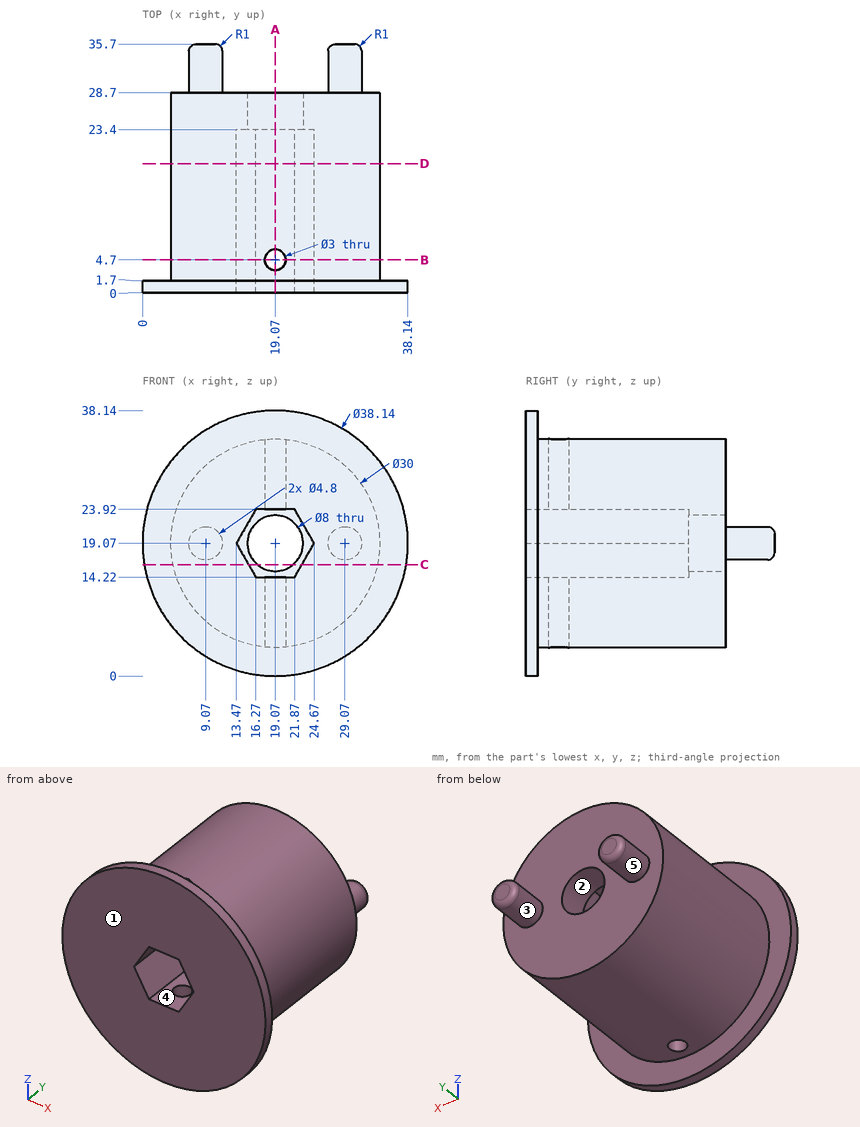
Study the drawing (mm; zero at the part's minimum x, y, z) and answer. A direction names the side the tool comes from. Give positions to 0.01 mm unless a question says otherwise; leave off trailing zeros. Write each loop counter-clockwise with the first axis right and the second up, starting at its lowest first coordinate (ties: lowest second). Pieces come first, ordered by that corner, then holes. Notation, with made-up numbers: (-40, -2) - (-8, -2) arc R27 ccw to (-8, 25) - close; hole circle Ø4 at (49, 26.25). An arc over 180 degrees is marked (long way). Use a Markdown table: item, result.
1. Find the intervals of material crossed by probe 1 along Y at (x, z) = (19, 9); probe 2 along Z at (x, y) = (18.5, 17); probe 3 along Y at (x, z) = (31, 22), in increasing order. Write a range as from..to.
Values follow:
| item | result |
|---|---|
| probe 1 | y = 0..3.2, 6.2..28.7 |
| probe 2 | z = 4.08..14.22, 23.92..34.06 |
| probe 3 | y = 0..28.7 |
2. Section C-C on z = 16 is taken. Write down the section's boundary in (x, y).
Values follow:
| item | result |
|---|---|
| outline | (0.25, 0) - (15.24, 0) - (15.24, 23.4) - (16.51, 23.4) - (16.51, 28.7) - (4.39, 28.7) - (4.39, 1.7) - (0.25, 1.7) - close; (21.63, 23.4) - (22.9, 23.4) - (22.9, 0) - (37.89, 0) - (37.89, 1.7) - (33.75, 1.7) - (33.75, 28.7) - (21.63, 28.7) - close |
3. Section A-A on x = 19.07 is taken. Write down the section's boundary in (y, z).
Values follow:
| item | result |
|---|---|
| outline | (0, 0) - (1.7, 0) - (1.7, 4.07) - (3.2, 4.07) - (3.2, 14.22) - (0, 14.22) - close; (0, 23.92) - (3.2, 23.92) - (3.2, 34.07) - (1.7, 34.07) - (1.7, 38.14) - (0, 38.14) - close; (6.2, 4.07) - (28.7, 4.07) - (28.7, 15.07) - (23.4, 15.07) - (23.4, 14.22) - (6.2, 14.22) - close; (6.2, 23.92) - (23.4, 23.92) - (23.4, 23.07) - (28.7, 23.07) - (28.7, 34.07) - (6.2, 34.07) - close |
4. Each of these flat-tipped pins is pushed along its axis until it touches: P1, Ø10, axis at x = 33, z = 30, coming from the -Y side; P2, Ø1.7, axis at x = 17.5, y = 11, coming from the -Z side; P3, Ø2.5, axis at x = 19.07, y = 4.7, coming from the -Z side; P4, Ø6, axis at x = 19.5, y = 29.5, coming from the +Z side. Where does it stop, or does it pass through?
Values follow:
| item | result |
|---|---|
| P1 | stops at y = 0 |
| P2 | stops at z = 4.09 |
| P3 | passes through |
| P4 | stops at z = 34.07 |
5. For a pull along Z with two mould halves and no side action, classify the marked faces 1, 2 and 3 as released by +Z, released by -Z, zero draft, split by the parting line, or undercut.
Values follow:
| item | result |
|---|---|
| face 1 | zero draft |
| face 2 | undercut |
| face 3 | split by the parting line |
6. Section B-B on y = 4.7 is taken. Write down the section's boundary in (x, z) (1 decimal), plus the area to 3 significant figures.
Values follow:
| item | result |
|---|---|
| outline | (13.5, 19.1) - (16.3, 23.9) - (17.6, 23.9) - (17.6, 34) arc R15 ccw to (17.6, 4.1) - (17.6, 14.2) - (16.3, 14.2) - close; (20.6, 4.1) arc R15 ccw to (20.6, 34) - (20.6, 23.9) - (21.9, 23.9) - (24.7, 19.1) - (21.9, 14.2) - (20.6, 14.2) - close |
| area | 565 mm² |
7. Section D-D on y = 18.5 is taken. Write down the section's boundary in (x, z).
Values follow:
| item | result |
|---|---|
| outline | circle Ø30 at (19.07, 19.07); hole (13.47, 19.07) - (16.27, 14.22) - (21.87, 14.22) - (24.67, 19.07) - (21.87, 23.92) - (16.27, 23.92) - close |
8. A tool of negligible diameter and unlimited length cuts with its end or side. For the marked faces 4 and 5, from which of +Z, -Z, +X, -X, +Y, -Y can it reach the whole face along a straight path? Write none if from no direction.
Values follow:
| item | result |
|---|---|
| face 4 | -Y |
| face 5 | +Y |
